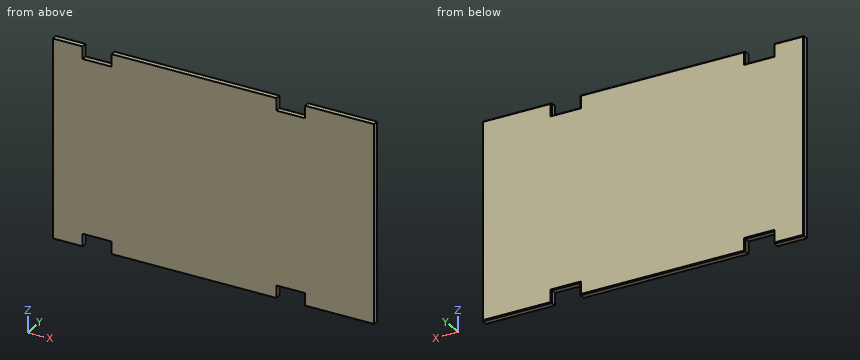
```python
from build123d import *

# Parameters (mm, degrees)
SKETCH1_W           = 990.6
SKETCH1_H           = 608.0125
BOSS_EXTRUDE1_DEPTH = 19.05
SKETCH2_W           = 88.9
SKETCH2_H           = 38.1
CUT_EXTRUDE1_DEPTH  = 20.05
CHAMFER1_SIZE       = 2.54


with BuildPart() as part:
    # Sketch1 → Boss-Extrude1 (new body)
    with BuildSketch(Plane(origin=(0, 0, 0), x_dir=(1, 0, 0), z_dir=(0, 1, 0))):
        with Locations((495.3, 304.00625)):
            Rectangle(SKETCH1_W, SKETCH1_H)
    extrude(amount=BOSS_EXTRUDE1_DEPTH)

    # Sketch2 → Cut-Extrude1 (cut, through all)
    with BuildSketch(Plane(origin=(0, 19.05, 0), x_dir=(1, 0, 0), z_dir=(0, 1, 0))):
        with Locations((733.425, 588.9625)):
            Rectangle(SKETCH2_W, SKETCH2_H)
        with Locations((136.525, 588.9625)):
            Rectangle(SKETCH2_W, SKETCH2_H)
        with Locations((136.525, 19.05)):
            Rectangle(SKETCH2_W, SKETCH2_H)
        with Locations((733.425, 19.05)):
            Rectangle(SKETCH2_W, SKETCH2_H)
    extrude(amount=-CUT_EXTRUDE1_DEPTH, mode=Mode.SUBTRACT)

    # Chamfer1
    chamfer1_edges = [part.edges().sort_by_distance(p)[0] for p in [
        (990.6, 19.05, -304.00625),
        (884.2375, 19.05, -608.0125),
        (434.975, 19.05, 0),
        (884.2375, 19.05, 0),
        (434.975, 19.05, -608.0125),
        (46.0375, 19.05, -608.0125),
        (733.425, 19.05, -38.1),
        (688.975, 19.05, -19.05),
        (777.875, 19.05, -19.05),
        (180.975, 19.05, -19.05),
        (136.525, 19.05, -38.1),
        (92.075, 19.05, -19.05),
        (92.075, 19.05, -588.9625),
        (136.525, 19.05, -569.9125),
        (180.975, 19.05, -588.9625),
        (0, 19.05, -304.00625),
        (777.875, 19.05, -588.9625),
        (688.975, 19.05, -588.9625),
        (733.425, 19.05, -569.9125),
        (46.0375, 19.05, 0),
    ]]
    chamfer(chamfer1_edges, length=CHAMFER1_SIZE)


solid = part.part
```
For this review, take the finished solid that the model builds, in its own axes (mm). Coordinates: 2 decimals unless noted, no trailing zeros. Loops run counter-clockwise (first coordinate to the right, second up) from the corner with the lowest first, then second, coordinate; pieces in that order, holes last.
1. Insertion check: P1, Ø5, axis at x = 449.5, z = -230.5, coming from the -Y side; P2, Ø8.5, axis at x = 734, y = 8.5, coming from the -Z side. Each pin has a flat end and moves straight along its axis. Give the tip position at first contact, or say it passes through.
2. Add section B-B, the plane x = 721.5. Give the boundary of the cut face in (y, z).
3. For line 1 (Z direction, x = 168, y = 16); line 2 (X direction, y = 18.25, z = -442.5); line 3 (Z direction, x = 128.5, y = 18), list the stretches that pass through material, from the lowest coordinate up.
4. Add section A-A, the plane y = 8.25. Give the boundary of the cut face in (x, z) (1 decimal).
Result:
1. P1: stops at y = 0
1. P2: stops at z = -569.91
2. outline: (0, -569.91) - (16.51, -569.91) - (19.05, -567.37) - (19.05, -40.64) - (16.51, -38.1) - (0, -38.1) - close
3. line 1: z = -569.91 to -38.1
3. line 2: x = 1.74 to 988.86
3. line 3: z = -568.42 to -39.59
4. outline: (0, -608) - (92.1, -608) - (92.1, -569.9) - (181, -569.9) - (181, -608) - (689, -608) - (689, -569.9) - (777.9, -569.9) - (777.9, -608) - (990.6, -608) - (990.6, 0) - (777.9, 0) - (777.9, -38.1) - (689, -38.1) - (689, 0) - (181, 0) - (181, -38.1) - (92.1, -38.1) - (92.1, 0) - (0, 0) - close
